from build123d import *

# Parameters (mm, degrees)
F0_R     = 254
F1_DEPTH = 76.2
F2_R     = 50.8
F3_SIZE  = 5.08
F4_R     = 114.7296539916
F5_DEPTH = 76.201
F6_R     = 38.1
F8_R     = 16.3985749671
F9_DEPTH = 388.62
F10_SIZE = 5.08


with BuildPart() as f1:
    # F0 (on Top) → F1 (new body)
    with BuildSketch(Plane.XY):
        Circle(F0_R)
    extrude(amount=F1_DEPTH)

    # F2
    f2_edges = [f1.edges().sort_by_distance(p)[0] for p in [
        (-254, 0, 76.2),
    ]]
    fillet(f2_edges, radius=F2_R)

    # F3
    f3_edges = [f1.edges().sort_by_distance(p)[0] for p in [
        (-254, 0, 0),
    ]]
    chamfer(f3_edges, length=F3_SIZE)

    # F4 (on face) → F5 (cut, through all)
    with BuildSketch(Plane.XY.offset(76.2)):
        Circle(F4_R)
    extrude(amount=-F5_DEPTH, mode=Mode.SUBTRACT)

    # F6 (on Front) → F7 (revolve, cut)
    with BuildSketch(Plane.XZ):
        with Locations((-156.143784523, 84.9872082472)):
            Circle(F6_R)
    revolve(axis=Axis((0, 0, 25.4), (0, 0, 1)), mode=Mode.SUBTRACT)

    # F8 (on Front) → F9 (cut, symmetric)
    with BuildSketch(Plane.XZ):
        with Locations((0, 77.1225020289)):
            Circle(F8_R)
    extrude(amount=F9_DEPTH, both=True, mode=Mode.SUBTRACT)

    # F10
    f10_edges = [f1.edges().sort_by_distance(p)[0] for p in [
        (-114.729654, 0, 0),
    ]]
    chamfer(f10_edges, length=F10_SIZE)


solid = f1.part
Can you work these out from the model? Positions are in its coordinate system, mm. Round coordinates to 2 decimals unless told otherwise and drop trailing zeros. Write each loop counter-clockwise with the first axis right and the second up, starting at its lowest first coordinate (ties: lowest second). Pieces come first, ordered by that corner, then holes. Notation, with made-up numbers: (54, 80) -> (58, 80) arc R9 ccw to (58, 84) -> close; hole circle Ø9 at (-17.75, 85). An arc over 180 degrees is marked (long way). Use one line per item in the form item = value. Start each with the question number.
Q1. I'm going to push flat-ended pins straight in: P1, Ø3, axis at y = 93, z = 36, coming from the +X side; P2, Ø12, axis at x = 154, y = -53.5, coming from the +Z side; P3, Ø1.5, axis at x = -54.5, z = 57, coming from the +Y side. Where does each tip first touch, or does it pass through?
Q2. We'd pull the mould along X, two halves only. Please class faces 1 (the face through (109.67, 34.54, 4.83)), 2 (the face through (-193, -14, 76.2)), 3 (the face through (237.661, 74.843, 0.247)): +X half, -X half, draft (parallel to the pull), parting line (faces both ways), or undercut.
Q3. Imagine slicing it at B-B (y = 0). Please give me the cut outline in (x, z).
Q4. If I drill on probe 1 along Y at (x, z) = (-99.5, 66); probe 2 along Y at (x, z) = (13.5, 29); probe 3 along X at (y, z) = (55, 34), over which ranges is the centre line in solid material (lowest first)? Write a range as [from, to].
Q5. Imagine slicing it at A-A (x = 0). Please give me the cut outline in (y, z), then the cut area to 3 significant figures.
Worked out:
q1.P1 = 235.84
q1.P2 = 49.13
q1.P3 = 237.41
q2.face_1 = undercut
q2.face_2 = draft
q2.face_3 = parting line
q3.outline = (-254, 5.08) -> (-248.92, 0) -> (-119.81, 0) -> (-114.73, 5.08) -> (-114.73, 76.2) -> (-119.07, 76.2) arc R38.1 cw to (-193.22, 76.2) -> (-203.2, 76.2) arc R50.8 ccw to (-254, 25.4) -> close; (114.73, 5.08) -> (119.81, 0) -> (248.92, 0) -> (254, 5.08) -> (254, 25.4) arc R50.8 ccw to (203.2, 76.2) -> (193.22, 76.2) arc R38.1 cw to (119.07, 76.2) -> (114.73, 76.2) -> close
q4.probe_1 = [-211.5, -160.89], [-72.5, -57.12], [57.12, 72.5], [160.89, 211.5]
q4.probe_2 = [-253.51, -113.93], [113.93, 253.51]
q4.probe_3 = [-247.22, -100.69], [100.69, 247.22]
q5.outline = (-254, 5.08) -> (-248.92, 0) -> (-119.81, 0) -> (-114.73, 5.08) -> (-114.73, 60.72) -> (-126.77, 60.72) arc R38.1 cw to (-185.52, 60.72) -> (-239.71, 60.72) arc R50.8 ccw to (-254, 25.4) -> close; (114.73, 5.08) -> (119.81, 0) -> (248.92, 0) -> (254, 5.08) -> (254, 25.4) arc R50.8 ccw to (239.71, 60.72) -> (185.52, 60.72) arc R38.1 cw to (126.77, 60.72) -> (114.73, 60.72) -> close
q5.area = 15,400 mm^2
